Can you work these out from the model? Positions are in its coordinate system, mm. A direction names the side the tool comes from. Coordinates: 2 decimals unless noted, no trailing zeros. Write each loop counter-clockwise with the first axis right and the second up, starting at its lowest first coordinate (ties: lowest second). Pieces come first, ordered by that corner, then holes. Notation, with made-up numbers: (-14.5, 43) -> (23.5, 43) arc R15 ccw to (23.5, 55) -> close; hole circle Ø1 at (-33, 58). An arc over 180 degrees is marked (long way). Use one line per item in the form item = value.
```python
from build123d import *

# Parameters (mm, degrees)
EXTRUDE_1_DEPTH     = 30
EXTRUDE_2_DEPTH     = 700
CUT_EXTRUDE_1_REACH = 1854.809


with BuildPart() as part:
    # Эскиз1 → Бобышка-Вытянуть1 (new body)
    with BuildSketch(Plane(origin=(0, 0, 0), x_dir=(1, 0, 0), z_dir=(0, 1, 0))):
        with BuildLine():
            Line((-1050, -650), (1050, -650))
            ThreePointArc((1050, -650), (1085.355339059, -635.355339059), (1100, -600))
            Line((1100, -600), (1100, 600))
            ThreePointArc((1100, 600), (1085.355339059, 635.355339059), (1050, 650))
            Line((1050, 650), (-1050, 650))
            ThreePointArc((-1050, 650), (-1085.355339059, 635.355339059), (-1100, 600))
            Line((-1100, 600), (-1100, -600))
            ThreePointArc((-1100, -600), (-1085.355339059, -635.355339059), (-1050, -650))
        make_face()
    extrude(amount=EXTRUDE_1_DEPTH)

    # Эскиз2 → Бобышка-Вытянуть2 (add)
    with BuildSketch(Plane(origin=(0, 30, 0), x_dir=(1, 0, 0), z_dir=(0, 1, 0))):
        with BuildLine():
            Line((-1050, -650), (1050, -650))
            ThreePointArc((1050, -650), (1085.355339059, -635.355339059), (1100, -600))
            Line((1100, -600), (1100, 600))
            ThreePointArc((1100, 600), (1085.355339059, 635.355339059), (1050, 650))
            Line((1050, 650), (-1050, 650))
            ThreePointArc((-1050, 650), (-1085.355339059, 635.355339059), (-1100, 600))
            Line((-1100, 600), (-1100, -600))
            ThreePointArc((-1100, -600), (-1085.355339059, -635.355339059), (-1050, -650))
        make_face()
        with BuildLine():
            Line((-1000, -600), (1000, -600))
            ThreePointArc((1000, -600), (1035.355339059, -585.355339059), (1050, -550))
            Line((1050, -550), (1050, 550))
            ThreePointArc((1050, 550), (1035.355339059, 585.355339059), (1000, 600))
            Line((1000, 600), (-1000, 600))
            ThreePointArc((-1000, 600), (-1035.355339059, 585.355339059), (-1050, 550))
            Line((-1050, 550), (-1050, -550))
            ThreePointArc((-1050, -550), (-1035.355339059, -585.355339059), (-1000, -600))
        make_face(mode=Mode.SUBTRACT)
    extrude(amount=EXTRUDE_2_DEPTH)

    # Эскиз3 → Вырез-Вытянуть1 (cut, up to next)
    with BuildSketch(Plane.XY.offset(650), mode=Mode.PRIVATE) as cut_extrude_1_sk1:
        Polygon((0, 730), (1300, 500.774925079), (1300, 730), (-1300, 730), (-1300, 500.774925079), align=None)
    cut_extrude_1_tool1 = extrude(cut_extrude_1_sk1.sketch, amount=-CUT_EXTRUDE_1_REACH, mode=Mode.PRIVATE) & part.part
    add(cut_extrude_1_tool1.solids().sort_by_distance((654.532365, 641.091783, 650))[0], mode=Mode.SUBTRACT)
    add(cut_extrude_1_tool1.solids().sort_by_distance((654.532365, 641.091783, 650))[1], mode=Mode.SUBTRACT)


solid = part.part
```
Q1. If I drill on line 1 (Z direction, x = -340, y = 536); line 2 (X direction, y = 483, z = -386); line 3 (Y direction, x = -289, z = -415.5), over which ranges is the centre line in solid material (lowest first)? Write a range as from..to.
Return value:
line_1 = -650..-600, 600..650
line_2 = -1100..-1050, 1050..1100
line_3 = 0..30
Q2. For faces 4 (the flat face through (-14, 375, 600)), 5 (the cylindrical face through (-1084.964, 268.614, -635.742)), which set-ups out of +Z, -Z, +X, -X, +Y, -Y let a thin tool reach every point of the face, with its end or its side?
Return value:
face_4 = +Y
face_5 = -Z, -X, +Y, -Y
Q3. Suppose I cut it at B-B (z = 146). Write out the boundary of the cut face in (x, y), then the cut area to 3 significant figures.
Return value:
outline = (-1100, 0) -> (1100, 0) -> (1100, 536.04) -> (1050, 544.86) -> (1050, 30) -> (-1050, 30) -> (-1050, 544.86) -> (-1100, 536.04) -> close
area = 117,000 mm2
Q4. Suppose I cut it at C-C (y = 466). Write out the boundary of the cut face in (x, z), then the cut area to 3 significant figures.
Return value:
outline = (-1100, -600) arc R50 ccw to (-1050, -650) -> (1050, -650) arc R50 ccw to (1100, -600) -> (1100, 600) arc R50 ccw to (1050, 650) -> (-1050, 650) arc R50 ccw to (-1100, 600) -> close; hole (-1050, -550) arc R50 ccw to (-1000, -600) -> (1000, -600) arc R50 ccw to (1050, -550) -> (1050, 550) arc R50 ccw to (1000, 600) -> (-1000, 600) arc R50 ccw to (-1050, 550) -> close
area = 340,000 mm2
Q5. Suppose I cut it at D-D (x = -826.5). Write out the boundary of the cut face in (y, z), then the cut area to 3 significant figures.
Return value:
outline = (0, -650) -> (584.27, -650) -> (584.27, -600) -> (30, -600) -> (30, 600) -> (584.27, 600) -> (584.27, 650) -> (0, 650) -> close
area = 94,400 mm2
Q6. Thinking about a two-plate mould opening in X: for faces 1 (the flat face through (1100, 264, 8)), 2 (the cylindrical face through (1035.742, 288.171, -584.964)), 3 (the flat face through (-15, 360, 650)), which applies, released by +X, released by -X, zero draft, split by the parting line, or undercut?
Return value:
face_1 = released by +X
face_2 = undercut
face_3 = zero draft
Q7. Suppose I cut it at A-A (y = 650.5). Write out the boundary of the cut face in (x, z), then the cut area to 3 significant figures.
Return value:
outline = (-450.87, -650) -> (450.87, -650) -> (450.87, -600) -> (-450.87, -600) -> close; (-450.87, 600) -> (450.87, 600) -> (450.87, 650) -> (-450.87, 650) -> close
area = 90,200 mm2
